Part model, mm, in its own coordinate system. A direction names the side the tool comes from. Round coordinates to 2 decimals unless told otherwise and drop trailing zeros. Loops run counter-clockwise (first coordinate to the right, second up) from the corner with the lowest first, then second, coordinate; pieces in that order, holes last. Notation, with made-up numbers: (-23.75, 52.25) - (20.25, 52.25) arc R13 ccw to (20.25, 63.25) - close; hole circle Ø6 at (62, 5.25). An arc over 180 degrees is marked (long way). Put each result on its own line as item: value.
from build123d import *

# Parameters (mm, degrees)
F1_DEPTH       = 34
F2_DEPTH       = 32
F0_R           = 1.5
F3_DEPTH       = 19
F4_R           = 12.5
F5_DEPTH       = 38
F7_W           = 25
F7_H           = 26
F8_DEPTH       = 32.4283063262
F9_R           = 20
F10_R          = 30
F11_R          = 1.99999
F12_R          = 20
F15_DEPTH      = 15
F15_DEPTH_BACK = 25
F16_R          = 2
F17_W          = 10
F17_H          = 6
F18_DEPTH      = 40
F19_R          = 1


# Not quite as in the source:
# - a fillet or chamfer is up to 0.001 mm smaller than in the source, because OpenCascade refuses the exact size


with BuildPart() as f1:
    # F0 (on Front) → F1 (new body, symmetric)
    with BuildSketch(Plane.XZ):
        with BuildLine():
            Line((90, -15), (90, 15))
            Line((90, 15), (-40, 15))
            Line((-40, 15), (-75, 15))
            Line((-75, 15), (-90, 0))
            Line((-90, 0), (-90, -15))
            Line((-90, -15), (-66.5, -15))
            ThreePointArc((-66.5, -15), (-66.4141111332, -12.9926634954), (-66.1570723538, -11))
            ThreePointArc((-66.1570723538, -11), (-43, 8.5), (-19.8429276462, -11))
            ThreePointArc((-19.8429276462, -11), (-19.5858888668, -12.9926634954), (-19.5, -15))
            Line((-19.5, -15), (19.5, -15))
            ThreePointArc((19.5, -15), (21.6186797268, -5.2486337688), (27.5926930532, 2.7444327226))
            ThreePointArc((27.5926930532, 2.7444327226), (37.7272727273, 13.516632815), (51.0436705831, 7.0805200018))
            ThreePointArc((51.0436705831, 7.0805200018), (62.2519642985, -1.5236551451), (66.5, -15))
            Line((66.5, -15), (90, -15))
        make_face()
        with BuildLine():
            ThreePointArc((27.5926930532, 2.7444327226), (38.7272727273, 8.1083059018), (51.0436705831, 7.0805200018))
            ThreePointArc((51.0436705831, 7.0805200018), (37.7272727273, 13.516632815), (27.5926930532, 2.7444327226))
        make_face()
    extrude(amount=F1_DEPTH, both=True)

    # F0 (on Front) → F2 (join, symmetric)
    with BuildSketch(Plane.XZ):
        Polygon((-40, 15), (90, 15), (0, 33.6523063262), align=None)
    extrude(amount=F2_DEPTH, both=True)

    # F0 (on Front) → F3 (join, symmetric)
    with BuildSketch(Plane.XZ):
        with BuildLine():
            Line((-66.5, -15), (-19.5, -15))
            ThreePointArc((-19.5, -15), (-19.5858888668, -12.9926634954), (-19.8429276462, -11))
            Line((-19.8429276462, -11), (-66.1570723538, -11))
            ThreePointArc((-66.1570723538, -11), (-66.4141111332, -12.9926634954), (-66.5, -15))
        make_face()
        with Locations((-43, -13)):
            Circle(F0_R, mode=Mode.SUBTRACT)
        with BuildLine():
            Line((19.5, -15), (66.5, -15))
            ThreePointArc((66.5, -15), (62.2519642985, -1.5236551451), (51.0436705831, 7.0805200018))
            ThreePointArc((51.0436705831, 7.0805200018), (52.1304551087, 4.2419425981), (52.5, 1.2249807396))
            ThreePointArc((52.5, 1.2249807396), (39.2388616534, -11.2518244772), (27.5926930532, 2.7444327226))
            ThreePointArc((27.5926930532, 2.7444327226), (21.6186797268, -5.2486337688), (19.5, -15))
        make_face()
        with Locations((43, -13)):
            Circle(F0_R, mode=Mode.SUBTRACT)
        with BuildLine():
            ThreePointArc((52.5, 1.2249807396), (52.1304551087, 4.2419425981), (51.0436705831, 7.0805200018))
            ThreePointArc((51.0436705831, 7.0805200018), (38.7272727273, 8.1083059018), (27.5926930532, 2.7444327226))
            ThreePointArc((27.5926930532, 2.7444327226), (39.2388616534, -11.2518244772), (52.5, 1.2249807396))
        make_face()
    extrude(amount=F3_DEPTH, both=True)

    # F4 (on face) → F5 (cut)
    with BuildSketch(Plane.XZ.offset(19)):
        with Locations((40, 1.2249807396)):
            Circle(F4_R)
    extrude(amount=-F5_DEPTH, mode=Mode.SUBTRACT)

    # F7 (on offset) → F8 (cut, through all)
    with BuildSketch(Plane.XY.offset(1.225)):
        with Locations((40, 6)):
            Rectangle(F7_W, F7_H)
    extrude(amount=F8_DEPTH, mode=Mode.SUBTRACT)

    # F9
    f9_edges = [f1.edges().sort_by_distance(p)[0] for p in [
        (0, 0, 33.652306),
        (-90, 0, 0),
    ]]
    fillet(f9_edges, radius=F9_R)

    # F10
    f10_edges = [f1.edges().sort_by_distance(p)[0] for p in [
        (-75, 0, 15),
    ]]
    fillet(f10_edges, radius=F10_R)

    # F11 (radius 2 in the source; OpenCascade refuses exactly that, so slightly less here)
    f11_edges = [f1.edges().sort_by_distance(p)[0] for p in [
        (13.713203, -34, 15),
        (13.713203, 34, 15),
    ]]
    fillet(f11_edges, radius=F11_R)

    # F12
    f12_edges = [f1.edges().sort_by_distance(p)[0] for p in [
        (90, 0, -15),
    ]]
    fillet(f12_edges, radius=F12_R)

    # F14 (on face) → F15 (join, two sides)
    with BuildSketch(Plane(origin=(45.8128559398, 0, -9.4946158074), x_dir=(0, 1, 0), z_dir=(0.9791921158, 0, -0.2029354588))) as f15_sk:
        Polygon((-32, 37.2520730314), (-32, 32.9520730314), (-30, 32.9520730314), (-30, 35.7520730314), (-28.5, 35.7520730314), (-28.5, 37.2520730314), align=None)
        Polygon((28.5, 35.7520730314), (30, 35.7520730314), (30, 32.9520730314), (32, 32.9520730314), (32, 37.2520730314), (28.5, 37.2520730314), align=None)
    extrude(amount=F15_DEPTH)
    extrude(f15_sk.sketch, amount=-F15_DEPTH_BACK)

    # F16
    f16_edges = [f1.edges().sort_by_distance(p)[0] for p in [
        (48.476662, -32, 27.996998),
        (48.476662, 32, 27.996998),
    ]]
    fillet(f16_edges, radius=F16_R)

    # F17 (on face) → F18 (cut)
    with BuildSketch(Plane(origin=(45.8128559398, 0, -9.4946158074), x_dir=(0, 1, 0), z_dir=(0.9791921158, 0, -0.2029354588))):
        with Locations((0, 32.9520730314)):
            Rectangle(F17_W, F17_H)
    extrude(amount=F18_DEPTH, mode=Mode.SUBTRACT)

    # F19
    f19_edges = [f1.edges().sort_by_distance(p)[0] for p in [
        (52.5, 0, 19.708044),
        (52.5, -5, 21.239919),
        (52.5, 5, 21.239919),
        (71.25, -5, 15.822147),
        (71.25, 5, 15.822147),
        (71.25, -5, 18.885897),
        (71.25, 5, 18.885897),
    ]]
    fillet(f19_edges, radius=F19_R)


solid = f1.part
1. Band-saw the part on A-A (y = 25.5). List the corners of the cut face in (x, z), plus the area to 3 significant figures.
A:
outline: (-90, -15) - (-66.5, -15) arc R23.5 cw to (-19.5, -15) - (19.5, -15) arc R23.5 cw to (66.5, -15) - (70, -15) arc R20 ccw to (90, 5) - (90, 15) - (6.5, 32.31) arc R20 ccw to (-6.01, 30.85) - (-40, 15) - (-62.57, 15) arc R30 ccw to (-83.79, 6.21) - (-84.14, 5.86) arc R20 ccw to (-90, -8.28) - close
area: 4,650 mm²
2. Pin check, flat tips, straight feed: P1, Ø19.5, axis at x = 24, z = 28, coming from the -Y side; P2, Ø1, axis at x = 69.5, y = 24.5, coming from the +Z side; P3, Ø5, axis at x = 43, z = -13, coming from the +Y side; P4, Ø11, axis at x = 44.5, z = -1.5, coming from the -Y side. Stop position of each tip, or through.
A:
P1: stops at y = -32
P2: stops at z = 19.35
P3: stops at y = 19
P4: passes through
3. Band-saw the part on B-B (x = 35). Give the number of separate pieces and of enclosed holes in the cut face, plus the area to 3 significant figures.
A:
separate pieces: 3
enclosed holes: 0
area: 898 mm²
4. Tool access for faces 4 (the flat face through (-43, 0, -11)), 5 (the flat face through (40, 19, 15)), 6 (the flat face through (24, 32, 22)), 7 (the flat face through (-43.3, 19, -11.2)): list every direction of +Z, -Z, +X, -X, +Y, -Y with a clear straight run to the whole face (end or side of a thin tool).
A:
face 4: +Y, -Y
face 5: +Z
face 6: +Z, +X, -X, +Y
face 7: -Z, +Y
5. Two-plate mould, pull along X, no slides. Class faces 1 (the flat face through (13, -32, 22)), 2 (the flat face through (48, -19, -9)), 3 (the cylindrical face through (-88.435, -0.448, -0.529)): pulls with the +X half, pulls with the -X half, needs draft (parallel to the pull), parting line crosses it, or undercut.
A:
face 1: needs draft
face 2: undercut
face 3: pulls with the -X half
6. Probe line 1 along Y through (x, z) = (37, 11.5); line 2 along X through (y, z) = (5.5, -10); line 3 along X through (y, z) = (18.5, 2). List the from-to ranges inside material, lowest first. Write a range as [from, to].
A:
line 1: y = [-34, -19], [19, 34]
line 2: x = [-90, -65.96], [-20.04, 34.5], [45.5, 83.23]
line 3: x = [-87.15, -59.22], [-26.78, 27.5], [52.5, 89.77]
